Build history of the part. All positions in model axes, mm. A direction names the side the tool comes from. Round coordinates to 2 decimals unless told otherwise and drop trailing zeros. Write each loop counter-clockwise with the first axis right and the second up, starting at its lowest first coordinate (ties: lowest second). Pieces come first, ordered by that corner, then holes. Notation, with made-up numbers: (45, 51) -> (73, 51) arc R27 cw to (73, 85) -> close; hole circle Ø9 at (41, 58.25). An arc over 180 degrees is marked (long way). Answer in a Markdown table with one row per item.
```python
from build123d import *

# Parameters (mm, degrees)
EXTRUDE_1_DEPTH     = 10
CUT_EXTRUDE_1_DEPTH = 3


with BuildPart() as part:
    # 草图1 → 凸台-拉伸1 (new body)
    with BuildSketch(Plane(origin=(0, 0, 0), x_dir=(1, 0, 0), z_dir=(0, 1, 0))):
        with BuildLine():
            Line((0, 0), (0, -60))
            Line((0, -60), (130, -60))
            Line((130, -60), (130, 0))
            ThreePointArc((130, 0), (65, 65), (0, 0))
        make_face()
    extrude(amount=EXTRUDE_1_DEPTH)

    # 草图2 → 切除-拉伸1 (cut)
    with BuildSketch(Plane(origin=(0, 10, 0), x_dir=(1, 0, 0), z_dir=(0, 1, 0))):
        Polygon((5.251262658, -15), (30, -39.748737342), (54.748737342, -15), (30, 9.748737342), align=None)
        Polygon((100, 9.748737342), (75.251262658, -15), (100, -39.748737342), (124.748737342, -15), align=None)
    extrude(amount=-CUT_EXTRUDE_1_DEPTH, mode=Mode.SUBTRACT)


solid = part.part
```
Q1. Which spindle directions (+Z, -Z, +X, -X, +Y, -Y) get a long thin tool onto all of the face, cutting with end or side? Do faces 5 (the flat face through (64, 5, 60)), 6 (the flat face through (42.2, 8.52, 27.55)). Say none if no direction does.
A:
| item | result |
|---|---|
| face 5 | +Z, +X, -X, +Y, -Y |
| face 6 | +Y |
Q2. Drop a flat-ended pin along its axis: P1, Ø2, axis at x = 68.5, y = 4.5, coming from the -Z side. Give the stop position or say it passes through.
A:
| item | result |
|---|---|
| P1 | z = -64.95 |
Q3. Saw through at D-D on z = 16.5. Write the cut outline in (x, y).
A:
| item | result |
|---|---|
| outline | (0, 0) -> (130, 0) -> (130, 10) -> (123.25, 10) -> (123.25, 7) -> (76.75, 7) -> (76.75, 10) -> (53.25, 10) -> (53.25, 7) -> (6.75, 7) -> (6.75, 10) -> (0, 10) -> close |
Q4. Two-plate mould, pull along X, no slides. Class faces 1 (the flat face through (0, 5, 30)), 2 (the cylindrical face through (66.429, 4.93, -64.984)), 3 (the flat face through (64, 0, -3)), 4 (the flat face through (112.55, 8.52, 2.8)): released by +X, released by -X, zero draft, split by the parting line, or undercut.
A:
| item | result |
|---|---|
| face 1 | released by -X |
| face 2 | split by the parting line |
| face 3 | zero draft |
| face 4 | undercut |
Q5. Saw through at A-A on y = 8.5. Write the cut outline in (x, z), plus the area to 3 significant figures.
A:
| item | result |
|---|---|
| outline | (0, 0) arc R65 ccw to (130, 0) -> (130, 60) -> (0, 60) -> close; hole (5.25, 15) -> (30, -9.75) -> (54.75, 15) -> (30, 39.75) -> close; hole (75.25, 15) -> (100, -9.75) -> (124.75, 15) -> (100, 39.75) -> close |
| area | 12,000 mm² |
Q6. Wall check: line 1 (Y direction, x = 38, z = 6); line 2 (Z direction, x = 43, y = 8); line 3 (Z direction, x = 13, y = 3). Give the ranges that are in metal, low to high. Write a range as [from, to].
A:
| item | result |
|---|---|
| line 1 | [0, 7] |
| line 2 | [-61.16, 3.25], [26.75, 60] |
| line 3 | [-39, 60] |
Q7. Saw through at C-C on z = 36. Write the cut outline in (x, y).
A:
| item | result |
|---|---|
| outline | (0, 0) -> (130, 0) -> (130, 10) -> (103.75, 10) -> (103.75, 7) -> (96.25, 7) -> (96.25, 10) -> (33.75, 10) -> (33.75, 7) -> (26.25, 7) -> (26.25, 10) -> (0, 10) -> close |
Q8. Saw through at B-B on x = 51. Write the cut outline in (y, z).
A:
| item | result |
|---|---|
| outline | (0, -63.47) -> (10, -63.47) -> (10, 11.25) -> (7, 11.25) -> (7, 18.75) -> (10, 18.75) -> (10, 60) -> (0, 60) -> close |
